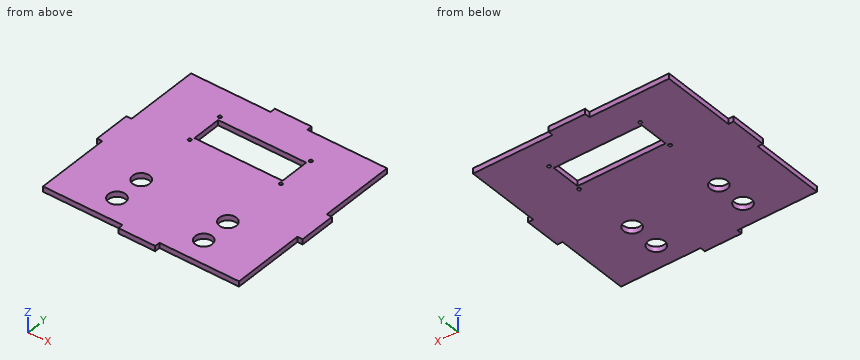
from build123d import *

# Parameters (mm, degrees)
SKETCH1_R           = 7
SKETCH1_R_2         = 1.35
SKETCH1_W           = 72.5
SKETCH1_H           = 24.5
BOSS_EXTRUDE1_DEPTH = 4.3


with BuildPart() as part:
    # Sketch1 → Boss-Extrude1 (new body)
    with BuildSketch(Plane.XY):
        Polygon((15.15, 76.515), (80.7, 76.515), (80.7, 14.135), (85, 14.135), (85, -16.165), (80.7, -16.165), (80.7, -76.515), (15.15, -76.515), (15.15, -80.815), (-15.15, -80.815), (-15.15, -76.515), (-80.7, -76.515), (-80.7, -15.15), (-85, -15.15), (-85, 15.15), (-80.7, 15.15), (-80.7, 76.515), (-15.15, 76.515), (-15.15, 80.815), (15.15, 80.815), align=None)
        with Locations(Location((35.7, -31.515, 0), (0, 0, 180))):
            Circle(SKETCH1_R, mode=Mode.SUBTRACT)
        with Locations(Location((35.7, -56.515, 0), (0, 0, 180))):
            Circle(SKETCH1_R, mode=Mode.SUBTRACT)
        with Locations(Location((-35.7, -56.515, 0), (0, 0, 180))):
            Circle(SKETCH1_R, mode=Mode.SUBTRACT)
        with Locations(Location((-35.7, -31.515, 0), (0, 0, 180))):
            Circle(SKETCH1_R, mode=Mode.SUBTRACT)
        with Locations(Location((-37.5, 52.015, 0), (0, 0, 180))):
            Circle(SKETCH1_R_2, mode=Mode.SUBTRACT)
        with Locations(Location((-37.5, 21.015, 0), (0, 0, 180))):
            Circle(SKETCH1_R_2, mode=Mode.SUBTRACT)
        with Locations(Location((37.5, 21.015, 0), (0, 0, 180))):
            Circle(SKETCH1_R_2, mode=Mode.SUBTRACT)
        with Locations(Location((37.5, 52.015, 0), (0, 0, 180))):
            Circle(SKETCH1_R_2, mode=Mode.SUBTRACT)
        with Locations((0, 36.515)):
            Rectangle(SKETCH1_W, SKETCH1_H, mode=Mode.SUBTRACT)
    extrude(amount=BOSS_EXTRUDE1_DEPTH)


solid = part.part
Input: part model. Units: mm. Frame: model coordinates. Give positions to 0.01 mm unless a question says otherwise; leave off trailing zeros. Order: outer loops, then holes, each group sorted by start corner. A loop starts at its lowest first (then second) coordinate and runs counter-clockwise, first axis right, second up.
Q1. Section C-C on z = 2.3. State how many separate pieces and enclosed holes the cut face has, and give its area (3 significant figures).
Checked values:
separate pieces: 1
enclosed holes: 9
area: 22,800 mm2
Q2. Contact query for flat-ended pins moving along their axis: pin 1 Ø2 at (x, z) = (63, 2.5) entering from +Y (3 decimals); pin 2 Ø1.3 at (y, z) = (-44, 2) entering from -X; pin 3 Ø1 at (y, z) = (-34, 1) entering from +X; pin 4 Ø11 at (x, y) = (35.7, -31.515) entering from -Z. Output: stop coordinate, or through.
Checked values:
pin 1: stops at y = 76.515
pin 2: stops at x = -80.7
pin 3: stops at x = 80.7
pin 4: passes through
Q3. Section B-B on y = 45. Output: boundary loops of the cut face in (x, z), and give its area (3 significant figures).
Checked values:
outline: (-80.7, 0) - (-36.25, 0) - (-36.25, 4.3) - (-80.7, 4.3) - close; (36.25, 0) - (80.7, 0) - (80.7, 4.3) - (36.25, 4.3) - close
area: 382 mm2
Q4. Section D-D on x = -53.5. Output: boundary loops of the cut face in (y, z) (3 decimals), and give its area (3 significant figures).
Checked values:
outline: (-76.515, 0) - (76.515, 0) - (76.515, 4.3) - (-76.515, 4.3) - close
area: 658 mm2
Q5. Section A-A on x = 18.5. Output: boundary loops of the cut face in (y, z) (3 decimals), and give its area (3 significant figures).
Checked values:
outline: (-76.515, 0) - (24.265, 0) - (24.265, 4.3) - (-76.515, 4.3) - close; (48.765, 0) - (76.515, 0) - (76.515, 4.3) - (48.765, 4.3) - close
area: 553 mm2
Q6. Ray query, probe 1 along Y at (x, z) = (35.7, 2.75) (3 decimals); probe 2 along Y at (x, z) = (18, 1) (3 decimals); probe 3 along X at (y, z) = (-51, 2.1). Return the intervals inside material, ascending.
Checked values:
probe 1: y = -76.515 to -63.515, -49.515 to -38.515, -24.515 to 24.265, 48.765 to 76.515
probe 2: y = -76.515 to 24.265, 48.765 to 76.515
probe 3: x = -80.7 to -40.01, -31.39 to 31.39, 40.01 to 80.7
